Input: part model. Units: mm. Frame: model coordinates. Face numbers are marked on the shaded views. Round coordinates to 2 decimals unless told otherwise and drop trailing zeros. Write each loop counter-clockwise with the first axis right and the second up, starting at its lowest first coordinate (ties: lowest second). Pieces come first, ordered by that corner, then holes. Notation, with made-up numbers: M -38,23 L 10,23 A22 ccw 10,53 Z; hole C -34,29.5 d9. An arc over 180 degrees is marked long. Write each question's results on one line, items separated by ' | '. Start each with the question number.
```python
from build123d import *

# Parameters (mm, degrees)
CUT_EXTRUDE1_DEPTH = 3.571875
CHAMFER1_SIZE      = 0.47625
CHAMFER2_SIZE      = 0.238125


with BuildPart() as part:
    # Sketch2 → Revolve1 (revolve)
    with BuildSketch(Plane(origin=(0, 0, 0), x_dir=(0, 0, -1), z_dir=(1, 0, 0)), mode=Mode.PRIVATE) as revolve1_sk:
        Polygon((12.7, 2.2225), (11.7475, 3.175), (-6.35, 3.175), (-6.35, 4.7625), (-12.7, 4.7625), (-12.7, 0), (12.7, 0), align=None)
    revolve(revolve1_sk.sketch.rotate(Axis((0, 0, -12.7), (0, 0, 1)), 90), axis=Axis((0, 0, -12.7), (0, 0, 1)))

    # Sketch4 → Cut-Extrude1 (cut)
    with BuildSketch(Plane.XY.offset(12.7)):
        Polygon((0, 2.749630657), (-2.38125, 1.374815329), (-2.38125, -1.374815329), (0, -2.749630657), (2.38125, -1.374815329), (2.38125, 1.374815329), align=None)
    extrude(amount=-CUT_EXTRUDE1_DEPTH, mode=Mode.SUBTRACT)

    # Cut-Extrude2 cone 1 section (on through the dimple's axis) → Cut-Extrude2 (revolve, cut)
    with BuildSketch(Plane(origin=(0, 0, 12.7), x_dir=(0, -1, 0), z_dir=(1, 0, 0))):
        Polygon((0, 0), (2.749630657, 0), (0, 1.5875), align=None)
    revolve(axis=Axis((0, 0, 12.7), (0, 0, -1)), mode=Mode.SUBTRACT)

    # Chamfer1
    chamfer1_edges = [part.edges().sort_by_distance(p)[0] for p in [
        (4.7625, 0, 12.7),
    ]]
    chamfer(chamfer1_edges, length=CHAMFER1_SIZE)

    # Chamfer2
    chamfer2_edges = [part.edges().sort_by_distance(p)[0] for p in [
        (4.7625, 0, 6.35),
    ]]
    chamfer(chamfer2_edges, length=CHAMFER2_SIZE)


solid = part.part
```
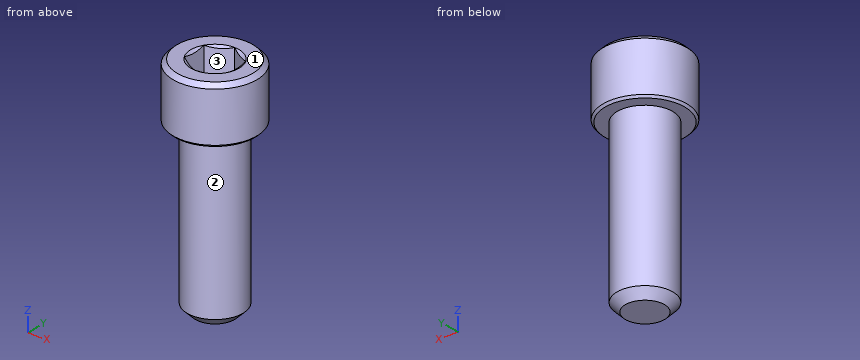
1. Draft query along X for the marked faces 1, 2 and 3. Return one class per face: +X half, -X half, draft (parallel to the pull), parting line (faces both ways), or undercut.
2. Line query: L1, parallel to Z at x = -2, y = 0; L2, parallel to Z at x = 3.5, y = 1.25; L3, parallel to Y at x = -1.25, z = 11.25. Output: solid intervals per line, ascending. Write a range as from..to.
3. Cut plane B-B on z = -2.5. Output: boundary loops of the cut face in (x, y) (3 decimals).
4. Contact query for flat-ended pins moving along their axis: P1, Ø4, axis at x = 1.5, z = -8.5, coming from the -Y side (3 decimals); P2, Ø3, axis at x = 3.5, z = -9, coming from the +Y side; P3, Ø4, axis at y = 1.5, z = 0.5, coming from the -X side (3 decimals). Output: stop coordinate, or through.
Answers follow:
1) face 1: draft | face 2: parting line | face 3: undercut
2) L1: z = -12.7..9.13 | L2: z = 6.35..12.7 | L3: y = -4.6..-2.03, 2.03..4.6
3) outline: C 0,0 d6.35
4) P1: stops at y = -3.175 | P2: stops at y = 2.47 | P3: stops at x = -3.175
